For this review, use the dimensioned drawing (mm, ordinates from the lowest corner) and the shaded views. A direction names the side the tool comes from. Coordinates: 2 decimals unless noted, no trailing zeros. Loops run counter-clockwise (first coordinate to the right, second up) from the corner with the lowest first, then second, coordinate; pieces in that order, holes last. Notation, with made-up numbers: M 46.25,42.5 L 55.25,42.5 A23 cw 55.25,54.5 Z; hole C 0,-27 d4. An arc over 180 degrees is marked long. One line per item, written item: value.
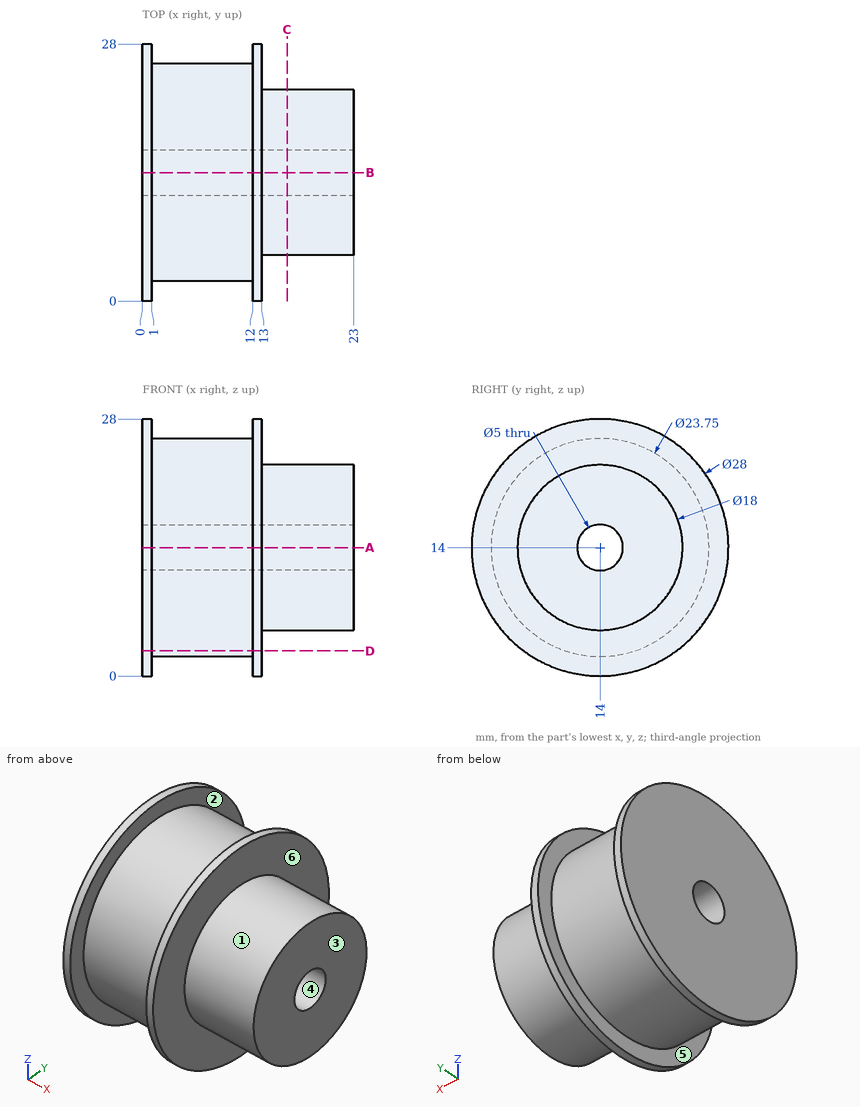
(1) We need section C-C on x = 15.75. State the section outline as (y, z) points, then the cut area to 3 significant figures.
Reply:
outline: C 14,14 d18; hole C 14,14 d5
area: 235 mm2
(2) We need section A-A on z = 14. State the section outline as (x, y) points (3 decimals).
Reply:
outline: M 0,0 L 1,0 L 1,2.125 L 12,2.125 L 12,0 L 13,0 L 13,5 L 23,5 L 23,11.5 L 0,11.5 Z; M 0,16.5 L 23,16.5 L 23,23 L 13,23 L 13,28 L 12,28 L 12,25.875 L 1,25.875 L 1,28 L 0,28 Z
(3) Mouldability with a two-part tool opening along X and no side actions: class the marked faces 1, 2 and 3 as released by +X, released by -X, zero draft, split by the parting line, or undercut.
Reply:
face 1: zero draft
face 2: undercut
face 3: released by +X
(4) To check wall thickness, follow line 1 along Y through (x, z) = (11.25, 14) (3 decimals); line 2 along X through (y, z) = (4.5, 5.5); line 3 along X through (y, z) = (15.75, 4). State the ranges of each line that lie inside material, in increasing order. Write a range as [from, to].
Reply:
line 1: y = [2.125, 11.5], [16.5, 25.875]
line 2: x = [0, 1], [12, 13]
line 3: x = [0, 13]
(5) Insertion check: pin 1 (8 mm diameter, centred on x = 6, z = 12, fed in from -Y) (3 decimals); pin 2 (4 mm diameter, centred on x = 11, y = 17.5, fed in from -Z); pin 3 (1 mm diameter, centred on x = 10, z = 17.5, fed in from +Y). Each pin has a flat end and moves straight along its axis. Give the tip position at first contact, or say it passes through.
Reply:
pin 1: stops at y = 2.125
pin 2: stops at z = 0.11
pin 3: stops at y = 25.49
(6) Tool access review of the marked faces 4, 5 and 6: name each direction out of +Z, -Z, +X, -X, +Y, -Y from which nothing blocks a thin tool from reaching the whole face with its end or side.
Reply:
face 4: +X, -X
face 5: none
face 6: +X
(7) We need section D-D on z = 2.75. State the section outline as (x, y) points.
Reply:
outline: M 0,5.67 L 1,5.67 L 1,10.2 L 12,10.2 L 12,5.67 L 13,5.67 L 13,22.33 L 12,22.33 L 12,17.8 L 1,17.8 L 1,22.33 L 0,22.33 Z
